CAD build for the part. Positions are in the model's coordinates, mm. Face numbers are marked on the shaded views. A direction names the side the tool comes from. Round coordinates to 2 decimals unless told otherwise and drop trailing zeros. Loops run counter-clockwise (first coordinate to the right, second up) from the corner with the lowest first, then second, coordinate; pieces in that order, holes last.
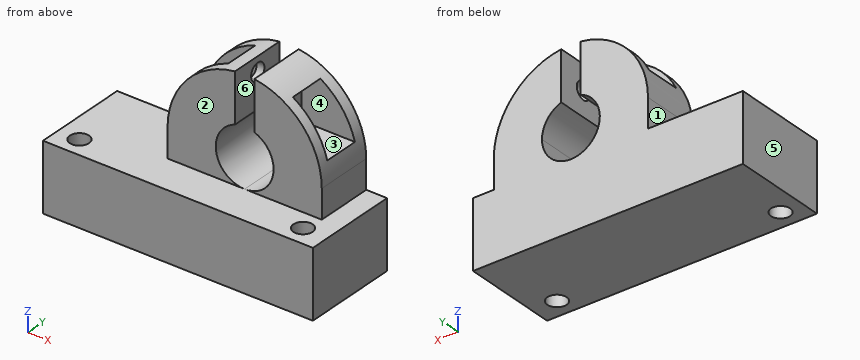
```python
from build123d import *

# Parameters (mm, degrees)
F1_DEPTH  = 50
F2_DEPTH  = 30
F3_R      = 4.5
F4_DEPTH  = 45.7741506228
F5_R      = 4.5
F6_DEPTH  = 84.2278493772
F7_R      = 5
F8_DEPTH  = 57
F9_W      = 18.3949293569
F9_H      = 20.3943792731
F10_DEPTH = 31
F11_W     = 18.6150614172
F11_H     = 23.8758381456
F12_DEPTH = 29


with BuildPart() as f1:
    # F0 (on Front) → F1 (new body)
    with BuildSketch(Plane.XZ):
        with BuildLine():
            Line((40, -15), (37.0809924355, -15))
            ThreePointArc((37.0809924355, -15), (0, -40), (-37.0809924355, -15))
            Line((-37.0809924355, -15), (-40, -15))
            Line((-40, -15), (-89.2268493772, -15))
            Line((-89.2268493772, -15), (-89.2268493772, -50))
            Line((-89.2268493772, -50), (50.7731506228, -50))
            Line((50.7731506228, -50), (50.7731506228, -15))
            Line((50.7731506228, -15), (40, -15))
        make_face()
        with BuildLine():
            Line((37.0809924355, -15), (0, -15))
            Line((0, -15), (-37.0809924355, -15))
            ThreePointArc((-37.0809924355, -15), (0, -40), (37.0809924355, -15))
        make_face()
    extrude(amount=F1_DEPTH)

    # F0 (on Front) → F2 (join)
    with BuildSketch(Plane.XZ):
        with BuildLine():
            Line((40, -15), (37.0809924355, -15))
            ThreePointArc((37.0809924355, -15), (0, -40), (-37.0809924355, -15))
            Line((-37.0809924355, -15), (-40, -15))
            Line((-40, -15), (-89.2268493772, -15))
            Line((-89.2268493772, -15), (-89.2268493772, -50))
            Line((-89.2268493772, -50), (50.7731506228, -50))
            Line((50.7731506228, -50), (50.7731506228, -15))
            Line((50.7731506228, -15), (40, -15))
        make_face()
        with BuildLine():
            Line((-37.0809924355, -15), (0, -15))
            ThreePointArc((0, -15), (-14.7839783948, -2.5365296809), (-5, 14.1421356237))
            Line((-5, 14.1421356237), (-5, 39.686269666))
            ThreePointArc((-5, 39.686269666), (-30, 26.4575131106), (-40, 0))
            ThreePointArc((-40, 0), (-39.2634671, -7.6406904983), (-37.0809924355, -15))
        make_face()
        with BuildLine():
            ThreePointArc((5, 14.1421356237), (12.2474487139, 8.6602540378), (15, 0))
            ThreePointArc((15, 0), (10.6066017178, -10.6066017178), (0, -15))
            Line((0, -15), (37.0809924355, -15))
            ThreePointArc((37.0809924355, -15), (39.2634671, -7.6406904983), (40, 0))
            ThreePointArc((40, 0), (30, 26.4575131106), (5, 39.686269666))
            Line((5, 39.686269666), (5, 14.1421356237))
        make_face()
        with BuildLine():
            Line((37.0809924355, -15), (0, -15))
            Line((0, -15), (-37.0809924355, -15))
            ThreePointArc((-37.0809924355, -15), (0, -40), (37.0809924355, -15))
        make_face()
        with BuildLine():
            Line((-40, -15), (-37.0809924355, -15))
            ThreePointArc((-37.0809924355, -15), (-39.2634671, -7.6406904983), (-40, 0))
            Line((-40, 0), (-40, -15))
        make_face()
        with BuildLine():
            ThreePointArc((40, 0), (39.2634671, -7.6406904983), (37.0809924355, -15))
            Line((37.0809924355, -15), (40, -15))
            Line((40, -15), (40, 0))
        make_face()
    extrude(amount=F2_DEPTH)

    # F3 (on face) → F4 (cut, through all)
    with BuildSketch(Plane(origin=(5, 0, 0), x_dir=(0, -1, 0), z_dir=(-1, 0, 0))):
        with Locations((15, 26.9142026448)):
            Circle(F3_R)
    extrude(amount=-F4_DEPTH, mode=Mode.SUBTRACT)

    # F5 (on face) → F6 (cut, through all)
    with BuildSketch(Plane.YZ.offset(-5)):
        with Locations((-14.6433338523, 32.090269666)):
            Circle(F5_R)
    extrude(amount=-F6_DEPTH, mode=Mode.SUBTRACT)

    # F7 (on face) → F8 (cut)
    with BuildSketch(Plane.XY.offset(-15)):
        with Locations((-78.0106559396, -40)):
            Circle(F7_R)
        with Locations((37.9573963583, -40)):
            Circle(F7_R)
    extrude(amount=-F8_DEPTH, mode=Mode.SUBTRACT)

    # F9 (on face) → F10 (cut)
    with BuildSketch(Plane(origin=(-40, 0, 0), x_dir=(0, -1, 0), z_dir=(-1, 0, 0))):
        with Locations((15.1999453083, 27.6889307424)):
            Rectangle(F9_W, F9_H)
    extrude(amount=-F10_DEPTH, mode=Mode.SUBTRACT)

    # F11 (on face) → F12 (cut)
    with BuildSketch(Plane.YZ.offset(40)):
        with Locations((-15.2023369446, 22.2436347976)):
            Rectangle(F11_W, F11_H)
    extrude(amount=-F12_DEPTH, mode=Mode.SUBTRACT)


solid = f1.part
```
Item 1: Flat gauge pins, fed straight in: P1, Ø10, axis at x = 32, z = -6.5, coming from the -Y side; P2, Ø2, axis at y = -29, z = -1.5, coming from the -X side; P3, Ø8, axis at y = -29.5, z = -6.5, coming from the +X side. Where does each tip first touch, or does it go through?
Answers follow:
P1: stops at y = -30
P2: stops at x = -40
P3: stops at x = 40
Item 2: Cut at A-A, the plane y = -40. Give the cut face in (x, z).
Answers follow:
outline: (-89.23, -50) - (-83.01, -50) - (-83.01, -15) - (-89.23, -15) - close; (-73.01, -50) - (32.96, -50) - (32.96, -15) - (-73.01, -15) - close; (42.96, -50) - (50.77, -50) - (50.77, -15) - (42.96, -15) - close
Item 3: Two-plate mould, pull along X, no slides. Class the marked faces 4, 5 and 6: released by +X, released by -X, zero draft, split by the parting line, or undercut.
Answers follow:
face 4: zero draft
face 5: released by -X
face 6: undercut
Item 4: Cut at D-D, the plane y = -15. Give the cut face in (x, z), plus the area to 3 significant figures.
Answers follow:
outline: (-89.23, -50) - (50.77, -50) - (50.77, -15) - (40, -15) - (40, 0) arc R40 ccw to (38.65, 10.31) - (11, 10.31) - (11, 22.41) - (5, 22.41) - (5, 14.14) arc R15 cw (long way) to (-5, 14.14) - (-5, 27.6) - (-9, 27.6) - (-9, 17.49) - (-35.97, 17.49) arc R40 ccw to (-40, 0) - (-40, -15) - (-89.23, -15) - close; (-12.83, 37.89) - (-9, 37.89) - (-9, 36.58) - (-5, 36.58) - (-5, 39.69) arc R40 ccw to start; (5, 31.41) - (11, 31.41) - (11, 34.18) - (20.78, 34.18) arc R40 ccw to (5, 39.69) - close
area: 6,680 mm2
Item 5: 3-axis set-ups, long thin cutter, end or side, ignore diameter. For the marked faces 1, 2 and 3: which of +Z, -Z, +X, -X, +Y, -Y reach the whole face in a straight line?
Answers follow:
face 1: +Z, -X, +Y, -Y
face 2: +Z, +X, -X, -Y
face 3: +X
Item 6: Probe line 1 (X direction, y = -39.5, z = -16.5); line 2 (Y direction, x = 20.5, z = 17.5); line 3 (X direction, y = -13, z = 22.5). List the from-to ranges inside material, lowest first.
Answers follow:
line 1: x = -89.23 to -82.99, -73.04 to 32.98, 42.93 to 50.77
line 2: y = -30 to -24.51, -5.89 to 0
line 3: x = -9 to -5, 5 to 11
Item 7: Cut at B-B, the plane z = -43. Give the cut face in (x, y), plus the area to 3 significant figures.
Answers follow:
outline: (-89.23, -50) - (50.77, -50) - (50.77, 0) - (-89.23, 0) - close; hole circle Ø10 at (-78.01, -40); hole circle Ø10 at (37.96, -40)
area: 6,840 mm2
Item 8: Cut at C-C, the plane z = -13.5. Give the cut face in (x, y).
Answers follow:
outline: (-40, -30) - (-6.54, -30) - (-6.54, 0) - (-40, 0) - close; (6.54, -30) - (40, -30) - (40, 0) - (6.54, 0) - close
